from build123d import *

# Parameters (mm, degrees)
F0_R     = 130.860579
F1_DEPTH = 100
F2_R     = 70
F3_DEPTH = 20
F4_W     = 309.986204
F4_H     = 334.951535
F5_DEPTH = 150


with BuildPart() as f1:
    # F0 (on Right) → F1 (new body)
    with BuildSketch(Plane.YZ):
        Circle(F0_R)
    extrude(amount=F1_DEPTH)

    # F2 (on face) → F3 (cut)
    with BuildSketch(Plane.YZ.offset(100)):
        with Locations((-9.41853, 0)):
            Circle(F2_R)
    extrude(amount=-F3_DEPTH, mode=Mode.SUBTRACT)

    # F4 (on Front) → F5 (cut)
    with BuildSketch(Plane.XZ):
        with Locations((44.957653, 2.534858)):
            Rectangle(F4_W, F4_H)
    extrude(amount=F5_DEPTH, mode=Mode.SUBTRACT)


solid = f1.part
Verification items for the finished model (mm, model axes). A direction names the side the tool comes from. Give positions to 0.01 mm unless a question says otherwise; leave off trailing zeros. Order: outer loops, then holes, each group sorted by start corner. A loop starts at its lowest first (then second) coordinate and runs counter-clockwise, first axis right, second up. Notation, with made-up numbers: M 7.5,-10 L 63.5,-10 A18 cw 63.5,5 Z; hole C -38.75,-6.75 d11. An arc over 180 degrees is marked long. Answer as a JSON object with one key per item and string values. Group by question number.
1) Cross-section at D-D (z = -59.5). Enter the section's corners in (x, y).
2) Cross-section at C-C (y = 97.5). Enter the section's corners in (x, z).
3) Access from +Z, -Z, +X, -X, +Y, -Y to the whole of each face (thin tool, end or side, straight path). Record for faces 4 (the face through (49, 0, 2)), 5 (the face through (90.14, 60.567, -1.407)).
4) Cross-section at B-B (x = 56). Enter the section's corners in (y, z), then the cut area to 3 significant figures.
5) Cross-section at A-A (z = 0). Enter the section's corners in (x, y).
6) Mould release check, pull along Z, two halves, no side actions. Record for faces 1 (the face through (49.3, 130.83, -2.88)), 2 (the face through (80, 23, 1)), 3 (the face through (0, 50, 2)): released by +Z, released by -Z, zero draft, split by the parting line, or undercut.
7) Scan lines: line 1 along Z through (x, y) = (87.5, 13.5); line 2 along Z through (x, y) = (95, 19.5); line 3 along Z through (x, y) = (23, 43). Record each from-to range of solid material in increasing order. Write a range as [from, to].
8) Depth check by flat-ended pin: pin 1 Ø6 at (x, y) = (74.5, 95.5) entering from -Z; pin 2 Ø2 at (x, z) = (86, -7.5) entering from +Y; pin 3 Ø2 at (x, z) = (36, -56) entering from +Y. Enter the tip coordinate at first touch or a pass-through.
Result sheet:
{
 "1": {"outline": "M 0,0 L 80,0 L 80,27.46 L 100,27.46 L 100,116.55 L 0,116.55 Z"},
 "2": {"outline": "M 0,-87.28 L 100,-87.28 L 100,87.28 L 0,87.28 Z"},
 "3": {"face 4": "+Z, -Z, +X, -X, -Y", "face 5": "+X, -Y"},
 "4": {"outline": "M 0,-130.86 A130.86 ccw 0,130.86 Z", "area": "26,900 mm2"},
 "5": {"outline": "M 0,0 L 80,0 L 80,60.58 L 100,60.58 L 100,130.86 L 0,130.86 Z"},
 "6": {"face 1": "split by the parting line", "face 2": "undercut", "face 3": "zero draft"},
 "7": {"line 1": "z = [-130.16, -66.14], [66.14, 130.16]", "line 2": "z = [-129.4, -63.75], [63.75, 129.4]", "line 3": "z = [-123.59, 123.59]"},
 "8": {"pin 1": "stops at z = -92.56", "pin 2": "stops at y = 130.7", "pin 3": "stops at y = 118.74"}
}
